Read the model definition and answer for the solid it produces. Units are mm, in the model's axes. A direction names the side the tool comes from. Coordinates: 2 decimals unless noted, no trailing zeros. Loops run counter-clockwise (first coordinate to the right, second up) from the corner with the lowest first, then second, coordinate; pieces in that order, holes last. Notation, with made-up numbers: (7.25, -39) -> (58.25, -39) arc R19 cw to (58.25, -10) -> close; hole circle Ø10 at (-36.75, 27). An arc over 180 degrees is marked (long way). Answer in a Markdown table with one row per item.
```python
from build123d import *

# Parameters (mm, degrees)
SKETCH1_W           = 250
SKETCH1_H           = 350.4
SKETCH1_R           = 2.1
SKETCH1_R_2         = 2.5
SKETCH1_R_3         = 1.59
SKETCH1_R_4         = 12.5
SKETCH1_W_2         = 33
SKETCH1_H_2         = 90
BOSS_EXTRUDE1_DEPTH = 5
SKETCH12_W          = 250
SKETCH12_H          = 5
CUT_EXTRUDE2_DEPTH  = 83
CUT_EXTRUDE3_DEPTH  = 6
SKETCH15_W          = 20.294476706
SKETCH15_H          = 22.5
SKETCH15_W_2        = 16.246360579
CUT_EXTRUDE4_DEPTH  = 10


with BuildPart() as part:
    # Sketch1 → Boss-Extrude1 (new body)
    with BuildSketch(Plane.XY):
        with Locations((125, -175.2)):
            Rectangle(SKETCH1_W, SKETCH1_H)
        with Locations((125, -45)):
            Circle(SKETCH1_R, mode=Mode.SUBTRACT)
        with Locations((125, -4)):
            Circle(SKETCH1_R, mode=Mode.SUBTRACT)
        with Locations((246, -119.5)):
            Circle(SKETCH1_R_2, mode=Mode.SUBTRACT)
        with Locations((246, -170.5)):
            Circle(SKETCH1_R_2, mode=Mode.SUBTRACT)
        with Locations((180.06, -129.375)):
            Circle(SKETCH1_R_3, mode=Mode.SUBTRACT)
        with Locations((180.06, -160.625)):
            Circle(SKETCH1_R_3, mode=Mode.SUBTRACT)
        with Locations((125, -24.5)):
            Circle(SKETCH1_R_4, mode=Mode.SUBTRACT)
        with Locations((141.96, -129.375)):
            Circle(SKETCH1_R_3, mode=Mode.SUBTRACT)
        with Locations((154.66, -129.375)):
            Circle(SKETCH1_R_3, mode=Mode.SUBTRACT)
        with Locations((167.36, -129.375)):
            Circle(SKETCH1_R_3, mode=Mode.SUBTRACT)
        with Locations((141.96, -160.625)):
            Circle(SKETCH1_R_3, mode=Mode.SUBTRACT)
        with Locations((154.66, -160.625)):
            Circle(SKETCH1_R_3, mode=Mode.SUBTRACT)
        with Locations((167.36, -160.625)):
            Circle(SKETCH1_R_3, mode=Mode.SUBTRACT)
        with Locations((82.64, -160.625)):
            Circle(SKETCH1_R_3, mode=Mode.SUBTRACT)
        with Locations((95.34, -160.625)):
            Circle(SKETCH1_R_3, mode=Mode.SUBTRACT)
        with Locations((108.04, -160.625)):
            Circle(SKETCH1_R_3, mode=Mode.SUBTRACT)
        with Locations((82.64, -129.375)):
            Circle(SKETCH1_R_3, mode=Mode.SUBTRACT)
        with Locations((95.34, -129.375)):
            Circle(SKETCH1_R_3, mode=Mode.SUBTRACT)
        with Locations((108.04, -129.375)):
            Circle(SKETCH1_R_3, mode=Mode.SUBTRACT)
        with Locations((69.94, -160.625)):
            Circle(SKETCH1_R_3, mode=Mode.SUBTRACT)
        with Locations((69.94, -129.375)):
            Circle(SKETCH1_R_3, mode=Mode.SUBTRACT)
        with Locations((4, -170.5)):
            Circle(SKETCH1_R_2, mode=Mode.SUBTRACT)
        with Locations((4, -119.5)):
            Circle(SKETCH1_R_2, mode=Mode.SUBTRACT)
        with Locations((202.56, -145)):
            Rectangle(SKETCH1_W_2, SKETCH1_H_2, mode=Mode.SUBTRACT)
        with BuildLine():
            Line((146.7225, -129.375), (146.7225, -149.054634918))
            ThreePointArc((146.7225, -149.054634918), (148.31, -149.140223925), (149.8975, -149.054634918))
            Line((149.8975, -149.054634918), (149.8975, -129.375))
            ThreePointArc((149.8975, -129.375), (148.31, -127.7875), (146.7225, -129.375))
        make_face(mode=Mode.SUBTRACT)
        with BuildLine():
            Line((159.42, -129.375), (159.42, -149.054634918))
            ThreePointArc((159.42, -149.054634918), (161.01, -149.140492925), (162.6, -149.054634918))
            Line((162.6, -149.054634918), (162.6, -129.375))
            ThreePointArc((162.6, -129.375), (161.01, -127.785), (159.42, -129.375))
        make_face(mode=Mode.SUBTRACT)
        with BuildLine():
            Line((172.12, -129.375), (172.12, -149.054634918))
            ThreePointArc((172.12, -149.054634918), (173.71, -149.140492925), (175.3, -149.054634918))
            Line((175.3, -149.054634918), (175.3, -129.375))
            ThreePointArc((175.3, -129.375), (173.71, -127.785), (172.12, -129.375))
        make_face(mode=Mode.SUBTRACT)
        with BuildLine():
            Line((146.7225, -160.625), (146.7225, -180.304634918))
            ThreePointArc((146.7225, -180.304634918), (148.31, -180.390223925), (149.8975, -180.304634918))
            Line((149.8975, -180.304634918), (149.8975, -160.625))
            ThreePointArc((149.8975, -160.625), (148.31, -159.0375), (146.7225, -160.625))
        make_face(mode=Mode.SUBTRACT)
        with BuildLine():
            Line((159.42, -160.625), (159.42, -180.304634918))
            ThreePointArc((159.42, -180.304634918), (161.01, -180.390492925), (162.6, -180.304634918))
            Line((162.6, -180.304634918), (162.6, -160.625))
            ThreePointArc((162.6, -160.625), (161.01, -159.035), (159.42, -160.625))
        make_face(mode=Mode.SUBTRACT)
        with BuildLine():
            Line((172.12, -160.625), (172.12, -180.304634918))
            ThreePointArc((172.12, -180.304634918), (173.71, -180.390492925), (175.3, -180.304634918))
            Line((175.3, -180.304634918), (175.3, -160.625))
            ThreePointArc((175.3, -160.625), (173.71, -159.035), (172.12, -160.625))
        make_face(mode=Mode.SUBTRACT)
        with BuildLine():
            Line((103.2775, -129.375), (103.2775, -149.054634918))
            ThreePointArc((103.2775, -149.054634918), (101.69, -150.642134918), (100.1025, -149.054634918))
            Line((100.1025, -149.054634918), (100.1025, -129.375))
            ThreePointArc((100.1025, -129.375), (101.69, -127.7875), (103.2775, -129.375))
        make_face(mode=Mode.SUBTRACT)
        with BuildLine():
            Line((90.58, -129.375), (90.58, -149.054634918))
            ThreePointArc((90.58, -149.054634918), (88.99, -150.644634918), (87.4, -149.054634918))
            Line((87.4, -149.054634918), (87.4, -129.375))
            ThreePointArc((87.4, -129.375), (88.99, -127.785), (90.58, -129.375))
        make_face(mode=Mode.SUBTRACT)
        with BuildLine():
            Line((77.88, -129.375), (77.88, -149.054634918))
            ThreePointArc((77.88, -149.054634918), (76.29, -150.644634918), (74.7, -149.054634918))
            Line((74.7, -149.054634918), (74.7, -129.375))
            ThreePointArc((74.7, -129.375), (76.29, -127.785), (77.88, -129.375))
        make_face(mode=Mode.SUBTRACT)
        with BuildLine():
            Line((103.2775, -160.625), (103.2775, -180.304634918))
            ThreePointArc((103.2775, -180.304634918), (101.69, -181.892134918), (100.1025, -180.304634918))
            Line((100.1025, -180.304634918), (100.1025, -160.625))
            ThreePointArc((100.1025, -160.625), (101.69, -159.0375), (103.2775, -160.625))
        make_face(mode=Mode.SUBTRACT)
        with BuildLine():
            Line((90.58, -160.625), (90.58, -180.304634918))
            ThreePointArc((90.58, -180.304634918), (88.99, -181.894634918), (87.4, -180.304634918))
            Line((87.4, -180.304634918), (87.4, -160.625))
            ThreePointArc((87.4, -160.625), (88.99, -159.035), (90.58, -160.625))
        make_face(mode=Mode.SUBTRACT)
        with BuildLine():
            Line((77.88, -160.625), (77.88, -180.304634918))
            ThreePointArc((77.88, -180.304634918), (76.29, -181.894634918), (74.7, -180.304634918))
            Line((74.7, -180.304634918), (74.7, -160.625))
            ThreePointArc((74.7, -160.625), (76.29, -159.035), (77.88, -160.625))
        make_face(mode=Mode.SUBTRACT)
        with Locations((47.44, -145)):
            Rectangle(SKETCH1_W_2, SKETCH1_H_2, mode=Mode.SUBTRACT)
    extrude(amount=BOSS_EXTRUDE1_DEPTH)

    # Sketch12 → Cut-Extrude2 (cut)
    with BuildSketch(Plane.XZ.offset(350.4)):
        with Locations((125, 2.5)):
            Rectangle(SKETCH12_W, SKETCH12_H)
    extrude(amount=-CUT_EXTRUDE2_DEPTH, mode=Mode.SUBTRACT)

    # Sketch13 → Cut-Extrude3 (cut, through all)
    with BuildSketch(Plane.XY.offset(5)):
        with BuildLine():
            Line((38.250392508, -85), (26.604338358, -85))
            Line((26.604338358, -85), (26.604338358, -113))
            Line((26.604338358, -113), (0, -113))
            Line((0, -113), (0, 0))
            Line((0, 0), (96.559911457, 0))
            ThreePointArc((96.559911457, 0), (89.789212828, -57.855339059), (38.250392508, -85))
        make_face()
        with BuildLine():
            Line((250, 0), (250, -113))
            Line((250, -113), (223.395661642, -113))
            Line((223.395661642, -113), (223.395661642, -85))
            Line((223.395661642, -85), (211.749607492, -85))
            ThreePointArc((211.749607492, -85), (160.210787172, -57.855339059), (153.440088543, 0))
            Line((153.440088543, 0), (250, 0))
        make_face()
        with BuildLine():
            Line((62.5, -227.4), (62.5, -350.4))
            Line((62.5, -350.4), (187.5, -350.4))
            Line((187.5, -350.4), (187.5, -227.4))
            ThreePointArc((187.5, -227.4), (125, -164.9), (62.5, -227.4))
        make_face()
    extrude(amount=-CUT_EXTRUDE3_DEPTH, mode=Mode.SUBTRACT)

    # Sketch15 → Cut-Extrude4 (cut)
    with BuildSketch(Plane.XY.offset(5)):
        with Locations((90.603154155, -11.25)):
            Rectangle(SKETCH15_W, SKETCH15_H)
        with Locations((157.372787781, -11.25)):
            Rectangle(SKETCH15_W_2, SKETCH15_H)
    extrude(amount=-CUT_EXTRUDE4_DEPTH, mode=Mode.SUBTRACT)


solid = part.part
```
1. A tool of negligible diameter and unlimited length cuts with its end or side. For faces 5 (the cylindrical face through (137, -21, 2)), 6 (the cylindrical face through (181.11, -199.87, 2.54)), from which of +Z, -Z, +X, -X, +Y, -Y can it reach the whole face along a straight path? Write none if from no direction.
A:
| item | result |
|---|---|
| face 5 | +Z, -Z |
| face 6 | +Z, -Z, -Y |
2. A cutting plane is placed at C-C on z = 2. Count the separate pieces of the cut face and the enclosed holes in it, and give its area (3 significant figures).
A:
| item | result |
|---|---|
| separate pieces | 1 |
| enclosed holes | 33 |
| area | 31,400 mm2 |
3. Given pin 1 Ø2.5 at (y, z) = (-16.5, 3.5) entering from +X; pin 2 Ø3 at (x, z) = (34.5, 2) entering from +Y, each flat-ended and moving along its own axis, determine where each tip first touches the part or whether it passes through.
A:
| item | result |
|---|---|
| pin 1 | stops at x = 149.25 |
| pin 2 | stops at y = -85 |
4. A cutting plane is placed at A-A on x = 215. Give the vertices of the cut face in (y, z).
A:
| item | result |
|---|---|
| outline | (-267.4, 0) -> (-190, 0) -> (-190, 5) -> (-267.4, 5) -> close; (-100, 0) -> (-85, 0) -> (-85, 5) -> (-100, 5) -> close |
5. A cutting plane is placed at B-B on y = -16.5. Give the vertices of the cut face in (x, z).
A:
| item | result |
|---|---|
| outline | (100.75, 0) -> (115.4, 0) -> (115.4, 5) -> (100.75, 5) -> close; (134.6, 0) -> (149.25, 0) -> (149.25, 5) -> (134.6, 5) -> close |
6. Find the intervals of material crossed by probe 1 along X at (y, z) = (-127.5, 3.9); probe 2 along Y at (x, z) = (141.96, 2.15) (3 decimals); probe 3 along X at (y, z) = (-105.5, 3.5), in increasing order.
A:
| item | result |
|---|---|
| probe 1 | x = 0 to 30.94, 63.94 to 186.06, 219.06 to 250 |
| probe 2 | y = -167.245 to -162.215, -159.035 to -130.965, -127.785 to 0 |
| probe 3 | x = 26.6 to 30.94, 63.94 to 186.06, 219.06 to 223.4 |
7. The mould has two halves that part along X. Classify faces 1 (the flat face through (123, -162, 0)), 2 (the cylindrical face through (82.928, -66.206, 2.535)), 3 (the cylindrical face through (168.044, -67.177, 2.535)), 4 (the cylindrical face through (69.252, -199.143, 2.535)): pulls with the +X half, pulls with the -X half, needs draft (parallel to the pull), parting line crosses it, or undercut.
A:
| item | result |
|---|---|
| face 1 | needs draft |
| face 2 | pulls with the -X half |
| face 3 | pulls with the +X half |
| face 4 | undercut |
